For this review, take the finished solid that the model builds, in its own axes (mm). A direction names the side the tool comes from. Round coordinates to 2 decimals unless told otherwise and drop trailing zeros. Write each loop counter-clockwise with the first axis right and the second up, starting at its lowest first coordinate (ties: lowest second). Pieces come first, ordered by that corner, then holes.
from build123d import *

# Parameters (mm, degrees)
F1_DEPTH = 25.4


with BuildPart() as f1:
    # F0 (on Front) → F1 (new body)
    with BuildSketch(Plane.XZ):
        with BuildLine():
            Line((88.9, 0), (139.7, 0))
            ThreePointArc((139.7, 0), (-137.288251, 25.846203), (130.136275, -50.8))
            Line((130.136275, -50.8), (72.955946, -50.8))
            ThreePointArc((72.955946, -50.8), (-26.621668, -84.82038), (-88.9, 0))
            Line((-88.9, 0), (88.9, 0))
        make_face()
        with BuildLine():
            ThreePointArc((-72.955946, 50.8), (0, 88.9), (72.955946, 50.8))
            Line((72.955946, 50.8), (-72.955946, 50.8))
        make_face(mode=Mode.SUBTRACT)
    extrude(amount=F1_DEPTH)


solid = f1.part
(1) For faces 1 (the face through (24, -13, 0)), 2 (the face through (1, -13, 50.8)), 3 (the face through (-2, 0, 2)), list the 3-axis set-ups (+Z, -Z, +X, -X, +Y, -Y) from which the entire face can be reached by the end or side of a thin tool; tool diameter is ignored.
Geometry check:
face 1: +X, +Y, -Y
face 2: +Y, -Y
face 3: +Z, -Z, +X, -X, +Y
(2) For line 1 along Z through (x, y) = (-6.5, -16.75); line 2 along Z through (x, y) = (-63, -1.5); line 3 along X through (y, z) = (-23.75, 72.5), list the stretches that pass through material, from the lowest coordinate up.
Geometry check:
line 1: z = -139.55 to -88.66, 0 to 50.8, 88.66 to 139.55
line 2: z = -124.69 to -62.72, 0 to 50.8, 62.72 to 124.69
line 3: x = -119.41 to -51.45, 51.45 to 119.41
(3) We need section B-B, the plane z = -64. Give the boundary of the cut face in (x, y).
Geometry check:
outline: (-124.18, -25.4) - (-61.7, -25.4) - (-61.7, 0) - (-124.18, 0) - close; (61.7, -25.4) - (124.18, -25.4) - (124.18, 0) - (61.7, 0) - close
(4) We need section A-A, the plane x = 0. Give the boundary of the cut face in (y, z), and give its area (3 significant figures).
Geometry check:
outline: (-25.4, -139.7) - (0, -139.7) - (0, -88.9) - (-25.4, -88.9) - close; (-25.4, 0) - (0, 0) - (0, 50.8) - (-25.4, 50.8) - close; (-25.4, 88.9) - (0, 88.9) - (0, 139.7) - (-25.4, 139.7) - close
area: 3,870 mm2
(5) For pin 1 Ø1 at (x, y) = (6.5, -3) entering from -Z; pin 2 Ø8 at (y, z) = (-9, 105.5) entering from -X; pin 3 Ø1 at (x, y) = (83.5, -17) entering from -Z, all flat-tipped, find the tip position at first contact; note any pin that passes through.
Geometry check:
pin 1: stops at z = -139.57
pin 2: stops at x = -95.99
pin 3: stops at z = -112.37
(6) We need section D-D, the plane x = -60.5. Give the boundary of the cut face in (y, z).
Geometry check:
outline: (-25.4, -125.92) - (0, -125.92) - (0, -65.14) - (-25.4, -65.14) - close; (-25.4, 0) - (0, 0) - (0, 50.8) - (-25.4, 50.8) - close; (-25.4, 65.14) - (0, 65.14) - (0, 125.92) - (-25.4, 125.92) - close
(7) We need section C-C, the plane y = -20. Give the boundary of the cut face in (x, z).
Geometry check:
outline: (-88.9, 0) - (139.7, 0) arc R139.7 ccw (long way) to (130.14, -50.8) - (72.96, -50.8) arc R88.9 cw to start; hole (-72.96, 50.8) - (72.96, 50.8) arc R88.9 ccw to start
(8) Mouldability with a two-part tool opening along Z and no side actions: class faces 4 (the face through (-1.2, -12.52, 88.89)), 5 (the face through (-136.102, -12.522, 31.503)), 6 (the face through (-2, -25.4, 2)), 7 (the face through (102, -13, -50.8)) as pulls with the +Z half, pulls with the -Z half, needs draft (parallel to the pull), parting line crosses it, or undercut.
Geometry check:
face 4: undercut
face 5: parting line crosses it
face 6: needs draft
face 7: undercut
